For this review, take the finished solid that the model builds, in its own axes (mm). A direction names the side the tool comes from. Give positions to 0.01 mm unless a question says otherwise; leave off trailing zeros. Order: outer loops, then holes, each group sorted by start corner. A loop starts at its lowest first (then second) coordinate and runs counter-clockwise, first axis right, second up. Notation, with made-up numbers: M 17,61.25 L 61,61.25 A13 ccw 61,65.25 Z; hole C 38,80.5 d4. An arc over 180 degrees is marked long. Use CSV: the item, a comma, the result in double quotes. Start each with the question number.
(1) Clearance check with flat-ended pins moving along their axes: P1, Ø0.6, axis at y = 1, z = -1, coming from the +X side; P2, Ø1.3, axis at x = -0.5, z = -1.5, coming from the -Y side; P3, Ø0.6, axis at x = 1, z = -1.5, coming from the -Y side. State where each tip first meets the part, or that it passes through.
(2) Tool access review of faces 1 (the face through (-0.343, -0.8, -0.8)), 2 (the face through (-1, 1, 0)), 3 (the face through (-0.195, -1.487, -4.302)): name each direction out of +Z, -Z, +X, -X, +Y, -Y from which nothing blocks a thin tool from reaching the whole face with its end or side.
(3) Consider section A-A (z = -4). Write out the cut boundary in (x, y).
(4) Wall thickness on L1, parallel to Y at x = 0.3, z = -0.75; L2, parallel to X at y = -0.55, z = -5; L3, parallel to Z at x = -1.8, y = 1.25: over which ranges is each line inside the solid? List them lowest first. Write a range as from..to.
```python
from build123d import *

# Parameters (mm, degrees)
CROSS_DEPTH       = 3.2
CIRPATTERN1_COUNT = 4
FILLET1_R         = 0.8


with BuildPart() as part:
    # Sketch1 → RevolveBase (revolve)
    with BuildSketch(Plane(origin=(0, 0, 0), x_dir=(0, 0, -1), z_dir=(1, 0, 0)), mode=Mode.PRIVATE) as revolvebase_sk:
        Polygon((0, 0), (0, 2.75), (0.2375, 2.75), (1.65, 1.3375), (1.65, 1.65), (6, 1.65), (6, 0), align=None)
    revolve(revolvebase_sk.sketch.rotate(Axis((0, 0, 0), (0, 0, -1)), 90), axis=Axis((0, 0, 0), (0, 0, -1)))

    # Sketch3 → Cross (cut)
    with BuildSketch(Plane.XY):
        with BuildLine():
            Line((-0.342946789, 0), (0.342946789, 0))
            Line((0.342946789, 0), (0.342946789, 1.562813968))
            ThreePointArc((0.342946789, 1.562813968), (0, 1.6), (-0.342946789, 1.562813968))
            Line((-0.342946789, 1.562813968), (-0.342946789, 0))
        make_face()
    cross = extrude(amount=-CROSS_DEPTH, mode=Mode.SUBTRACT)

    # CirPattern1: Cross ×4 about axis
    cirpattern1_axis = Axis((0, 0, 0), (0, 0, 1))
    for i in range(1, CIRPATTERN1_COUNT):
        add(cross.rotate(cirpattern1_axis, i * 360 / CIRPATTERN1_COUNT), mode=Mode.SUBTRACT)

    # Sketch5 → RevolveRod (revolve)
    with BuildSketch(Plane(origin=(0, 0, 0), x_dir=(0, 0, -1), z_dir=(1, 0, 0)), mode=Mode.PRIVATE) as revolverod_sk:
        Polygon((0, 2.102030651), (0, 1.6), (1.935490568, 0.635), (2.273126058, 0), (6, 0), (6, 1.5), (1.65, 1.5), (1.65, 1.3375), (0.885469349, 2.102030651), align=None)
    revolve(revolverod_sk.sketch.rotate(Axis((0, 0, 0), (0, 0, -1)), 90), axis=Axis((0, 0, 0), (0, 0, -1)))

    # Sketch7 → CutBody (revolve, cut)
    with BuildSketch(Plane(origin=(0, 0, 0), x_dir=(0, 0, -1), z_dir=(1, 0, 0)), mode=Mode.PRIVATE) as cutbody_sk:
        Polygon((1.65, 3.5), (1.65, 1.3375), (2.65, 1.5), (6, 1.5), (6, 3.5), align=None)
    revolve(cutbody_sk.sketch.rotate(Axis((0, 0, 0), (0, 0, -1)), 90), axis=Axis((0, 0, 0), (0, 0, -1)), mode=Mode.SUBTRACT)

    # Fillet1
    fillet1_edges = [part.edges().sort_by_distance(p)[0] for p in [
        (1.326274207, -0.172924772, -1.65),
    ]]
    fillet(fillet1_edges, radius=FILLET1_R)


solid = part.part
```
Check result:
1,P1,"stops at x = 2.08"
1,P2,"stops at y = -2.09"
1,P3,"stops at y = -1.53"
2,face 1,"+Z"
2,face 2,"+Z, +X, -X, +Y, -Y"
2,face 3,"-Z"
3,outline,"C 0,0 d3"
4,L1,"y = -2.22..-1.19, 1.19..2.22"
4,L2,"x = -1.4..1.4"
4,L3,"z = -0.8..0"
